Build history of the part. All positions in model axes, mm. A direction names the side the tool comes from. Give positions to 0.01 mm unless a question says otherwise; leave off trailing zeros. Order: outer loops, then holes, each group sorted by start corner. A loop starts at its lowest first (then second) coordinate and runs counter-clockwise, first axis right, second up. Notation, with made-up numbers: (85, 29.25) - (135, 29.25) arc R23 ccw to (135, 42.25) - close; hole circle Ø7 at (-6.5, 63). An arc over 180 degrees is marked (long way). One line per item, written item: value.
```python
from build123d import *

# Parameters (mm, degrees)
BOSS_EXTRUDE1_DEPTH = 12.7
SKETCH2_W           = 34.925
SKETCH2_H           = 12.7
CUT_EXTRUDE1_DEPTH  = 619.139151001
SKETCH2_4_R         = 3.175
CUT_EXTRUDE2_DEPTH  = 6.35
SKETCH3_W           = 679.915177356
SKETCH3_H           = 6.35
CUT_EXTRUDE3_DEPTH  = 6.35


with BuildPart() as part:
    # Sketch1 → Boss-Extrude1 (new body)
    with BuildSketch(Plane.XY):
        Polygon((609.6, 88.9), (596.9, 88.9), (596.9, 76.2), (609.6, 76.2), (609.6, 63.5), (596.9, 63.5), (596.9, 50.8), (609.6, 50.8), (609.6, 38.1), (596.9, 38.1), (596.9, 25.4), (609.6, 25.4), (609.6, 12.7), (596.9, 12.7), (596.9, 0), (12.7, 0), (12.7, 12.7), (0, 12.7), (0, 25.4), (12.7, 25.4), (12.7, 38.1), (0, 38.1), (0, 50.8), (12.7, 50.8), (12.7, 63.5), (0, 63.5), (0, 76.2), (12.7, 76.2), (12.7, 88.9), (0, 88.9), (0, 101.6), (609.6, 101.6), align=None)
    extrude(amount=BOSS_EXTRUDE1_DEPTH)

    # Sketch2 → Cut-Extrude1 (cut, through all)
    with BuildSketch(Plane.XY):
        with Locations((579.4375, 6.35)):
            Rectangle(SKETCH2_W, SKETCH2_H)
        with Locations((30.1625, 6.35)):
            Rectangle(SKETCH2_W, SKETCH2_H)
    extrude(amount=CUT_EXTRUDE1_DEPTH, mode=Mode.SUBTRACT)

    # Sketch2_4 → Cut-Extrude2 (cut)
    with BuildSketch(Plane.XY):
        with Locations((589.75625, 23.8125)):
            Circle(SKETCH2_4_R)
        with Locations((19.84375, 23.8125)):
            Circle(SKETCH2_4_R)
    extrude(amount=CUT_EXTRUDE2_DEPTH, mode=Mode.SUBTRACT)

    # Sketch3 → Cut-Extrude3 (cut)
    with BuildSketch(Plane.XY.offset(12.7)):
        with Locations((325.163434952, 15.875)):
            Rectangle(SKETCH3_W, SKETCH3_H)
    extrude(amount=-CUT_EXTRUDE3_DEPTH, mode=Mode.SUBTRACT)


solid = part.part
```
(1) Pull direction Y, two halves, no side cores. Call faces 1 (the face through (0, 20, 5)), 2 (the face through (6, 50.8, 6)), 3 (the face through (308, 0, 6)): +Y half, -Y half, draft (parallel to the pull), parting line (faces both ways), or undercut.
Completed:
face 1: draft
face 2: undercut
face 3: -Y half
(2) Slice it at C-C, the plane y = 82.5. Give the cut face in (x, z), and give its area (3 significant figures).
Completed:
outline: (12.7, 0) - (596.9, 0) - (596.9, 12.7) - (12.7, 12.7) - close
area: 7,420 mm²
(3) Drill centre lines: line 1 (Y direction, x = 292, z = 7.5); line 2 (X direction, y = 84, z = 6.25); line 3 (X direction, y = 11, z = 8) (3 decimals). Where is each one in solid material? Low to high.
Completed:
line 1: 0 to 12.7, 19.05 to 101.6
line 2: 12.7 to 596.9
line 3: 47.625 to 561.975
(4) Slice it at A-A, the plane x = 488.5. Give the cut face in (y, z), and give its area (3 significant figures).
Completed:
outline: (0, 0) - (101.6, 0) - (101.6, 12.7) - (19.05, 12.7) - (19.05, 6.35) - (12.7, 6.35) - (12.7, 12.7) - (0, 12.7) - close
area: 1,250 mm²
(5) Slice it at B-B, the plane z = 3.75. Count the separate pieces of the cut face and the enclosed holes in it, and give its area (3 significant figures).
Completed:
separate pieces: 1
enclosed holes: 2
area: 59,700 mm²
(6) Pin check, flat tips, straight feed: P1, Ø4, axis at y = 28.5, z = 9, coming from the +X side; P2, Ø1.9, axis at x = 31, z = 4.5, coming from the -Y side; P3, Ø1.9, axis at x = 21, y = 25, coming from the -Z side. Stop position of each tip, or through.
Completed:
P1: x = 596.9
P2: y = 12.7
P3: z = 6.35
(7) 3-axis set-ups, long thin cutter, end or side, ignore diameter. For faces 4 (the face through (561.975, 6, 6)), 5 (the face through (12.7, 82, 6)), 6 (the face through (596.9, 32, 6)): which of +Z, -Z, +X, -X, +Y, -Y reach the whole face in a straight line?
Completed:
face 4: +Z, -Z, +X, -Y
face 5: +Z, -Z, -X
face 6: +Z, -Z, +X
